Input: part model. Units: mm. Frame: model coordinates. Give positions to 0.01 mm unless a question says otherwise; leave off trailing zeros. Loops run counter-clockwise (first coordinate to the right, second up) from the corner with the lowest first, then second, coordinate; pieces in that order, holes last.
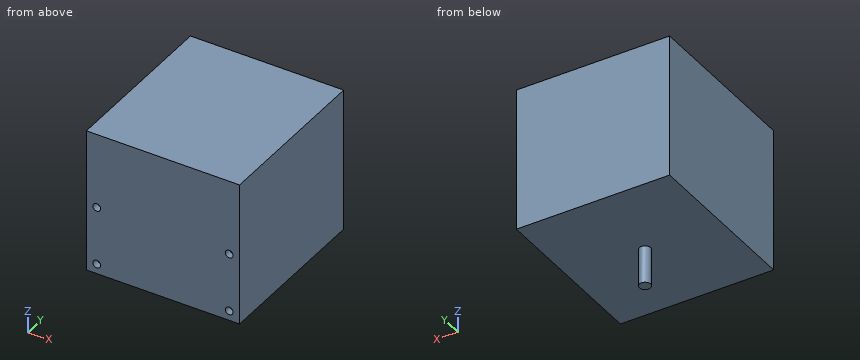
from build123d import *

# Parameters (mm, degrees)
BOSS_EXTRUDE1_DEPTH      = 4.978866735
BOSS_EXTRUDE1_DEPTH_BACK = 104.997590598
SKETCH1_W                = 119.988
SKETCH1_H                = 129.794
SKETCH3_OUTSIDE_W        = 153.613
SKETCH3_OUTSIDE_H        = 163.624
SKETCH3_OUTSIDE_R        = 4
CUT_EXTRUDE1_DEPTH       = 26.924
SKETCH4_R                = 2.8
CUT_EXTRUDE2_DEPTH       = 5


with BuildPart() as part:
    # Sketch1 → Boss-Extrude1 (new, two sides: drawn at the far end of the back side and taken through both)
    with BuildSketch(Plane.YZ.offset(-BOSS_EXTRUDE1_DEPTH_BACK)):
        with Locations((59.994, 64.897)):
            Rectangle(SKETCH1_W, SKETCH1_H)
    extrude(amount=BOSS_EXTRUDE1_DEPTH + BOSS_EXTRUDE1_DEPTH_BACK)

    # Sketch3 outside → Cut-Extrude1 (cut)
    with BuildSketch(Plane(origin=(0, 0, 0), x_dir=(1, 0, 0), z_dir=(0, 0, -1))):
        with Locations((-50.0095, -59.994)):
            Rectangle(SKETCH3_OUTSIDE_W, SKETCH3_OUTSIDE_H)
        with Locations(Location((-50.038, -59.994, 0), (0, 0, 180))):
            Circle(SKETCH3_OUTSIDE_R, mode=Mode.SUBTRACT)
    extrude(amount=-CUT_EXTRUDE1_DEPTH, mode=Mode.SUBTRACT)

    # Sketch4 → Cut-Extrude2 (cut)
    with BuildSketch(Plane.XZ):
        with Locations(Location((-97.538, 33.924, 0), (0, 0, 270))):
            Circle(SKETCH4_R)
        with Locations(Location((-97.538, 75.924, 0), (0, 0, 270))):
            Circle(SKETCH4_R)
        with Locations(Location((-2.480723862, 75.924, 0), (0, 0, 270))):
            Circle(SKETCH4_R)
        with Locations(Location((-2.480723862, 33.924, 0), (0, 0, 270))):
            Circle(SKETCH4_R)
    extrude(amount=-CUT_EXTRUDE2_DEPTH, mode=Mode.SUBTRACT)


solid = part.part
(1) Ray query, probe 1 along Z at (x, y) = (-6.5, 6). Return the intervals inside material, ascending.
Values follow:
probe 1: z = 26.92 to 129.79
(2) Pin query (flat end, axial travel): pin 1 Ø1 at (x, y) = (-55, 99.5) entering from -Z; pin 2 Ø3 at (x, z) = (-1.5, 75.5) entering from -Y; pin 3 Ø6 at (y, z) = (57.5, 17.5) entering from -X. Return the tip coordinate at first contact, or that it passes through.
Values follow:
pin 1: stops at z = 26.92
pin 2: stops at y = 5
pin 3: stops at x = -54.04
(3) Cut plane A-A (y = 86.5). Return the cut outline in (x, z), and give its area (3 significant figures).
Values follow:
outline: (-105, 26.92) - (4.98, 26.92) - (4.98, 129.79) - (-105, 129.79) - close
area: 11,300 mm2
(4) Cut plane B-B (x = -33.5). Return the cut outline in (y, z).
Values follow:
outline: (0, 26.92) - (119.99, 26.92) - (119.99, 129.79) - (0, 129.79) - close
(5) Cut plane C-C (z = 20.5). Return the cut outline in (x, y), and give its area (3 significant figures).
Values follow:
outline: circle Ø8 at (-50.04, 59.99)
area: 50.3 mm2
